Work out the finished part from the listing and answer in its coordinate system (mm). Face numbers are marked on the shaded views. A direction names the side the tool comes from. Coordinates: 2 decimals unless noted, no trailing zeros. Loops run counter-clockwise (first coordinate to the right, second up) from the corner with the lowest first, then second, coordinate; pieces in that order, holes last. Notation, with made-up numbers: M -27,75.25 L 7,75.25 A25 cw 7,112.25 Z; hole C 57.25,72 d4. An arc over 180 degrees is marked long. Write each question's results on one line, items separated by ' | '.
```python
from build123d import *

# Parameters (mm, degrees)
BOSS_EXTRUDE1_DEPTH     = 21
SKETCH3_R               = 14.5
BOSS_EXTRUDE2_DEPTH     = 16
CUT_EXTRUDE1_DEPTH      = 30.351320243
CUT_EXTRUDE1_DEPTH_BACK = 30.351320243
SKETCH4_R               = 5


with BuildPart() as part:
    # Sketch1 → Boss-Extrude1 (new body)
    with BuildSketch(Plane.XY):
        with BuildLine():
            Line((-8, 7.549834435), (-8, -7.549834435))
            ThreePointArc((-8, -7.549834435), (0, -11), (8, -7.549834435))
            Line((8, -7.549834435), (8, 7.549834435))
            ThreePointArc((8, 7.549834435), (0, 11), (-8, 7.549834435))
        make_face()
    extrude(amount=BOSS_EXTRUDE1_DEPTH)

    # Sketch3 → Boss-Extrude2 (add)
    with BuildSketch(Plane.XY):
        Circle(SKETCH3_R)
    extrude(amount=-BOSS_EXTRUDE2_DEPTH)

    # Sketch4 → Cut-Extrude1 (cut, two sides: drawn at the far end of the back side and taken through both)
    with BuildSketch(Plane(origin=(0, 0, 0), x_dir=(0, 0, -1), z_dir=(1, 0, 0)).offset(-CUT_EXTRUDE1_DEPTH_BACK)):
        with Locations((-11.179145377, 0)):
            Circle(SKETCH4_R)
    extrude(amount=CUT_EXTRUDE1_DEPTH + CUT_EXTRUDE1_DEPTH_BACK, mode=Mode.SUBTRACT)


solid = part.part
```
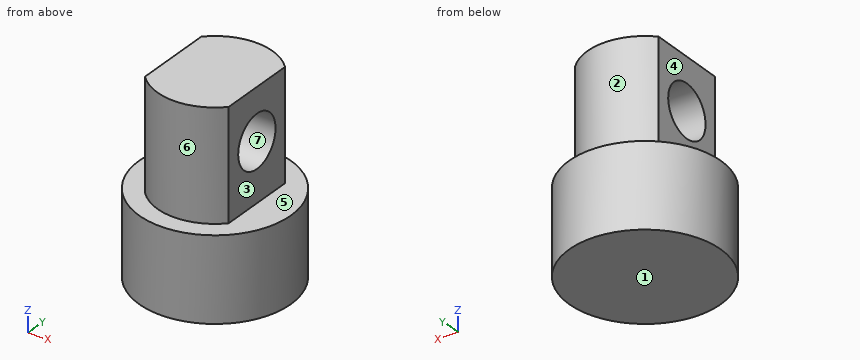
1) Find section D-D, the plane y = -4.25. Give the vertices of the cut face in (x, z).
Check result:
outline: M -13.86,-16 L 13.86,-16 L 13.86,0 L 8,0 L 8,8.55 L -8,8.55 L -8,0 L -13.86,0 Z; M -8,13.81 L 8,13.81 L 8,21 L -8,21 Z
2) For a pull along Z with two mould halves and no side action, classify the marked faces 5, 6 and 7 as released by +Z, released by -Z, zero draft, split by the parting line, or undercut.
Check result:
face 5: released by +Z | face 6: zero draft | face 7: undercut
3) Find section A-A, the plane y = 0. Give the vertices of the cut face in (x, z).
Check result:
outline: M -14.5,-16 L 14.5,-16 L 14.5,0 L 8,0 L 8,6.18 L -8,6.18 L -8,0 L -14.5,0 Z; M -8,16.18 L 8,16.18 L 8,21 L -8,21 Z
4) Find section C-C, the plane x = 0. Give the vertices of the cut face in (y, z).
Check result:
outline: M -14.5,-16 L 14.5,-16 L 14.5,0 L 11,0 L 11,21 L -11,21 L -11,0 L -14.5,0 Z; hole C 0,11.18 d10
5) Given pin 1 Ø16.5 at (y, z) = (1.5, 5.5) entering from -X; pin 2 Ø8 at (x, z) = (-10.5, -11.5) entering from +Y; pin 3 Ø13 at (y, z) = (0, 11.18) entering from +X; pin 4 Ø6 at (y, z) = (-6, 5.5) entering from -X, each flat-ended and moving along its own axis, determine where each tip first touches the part or whether it passes through.
Check result:
pin 1: x = -14.5 | pin 2: y = 12.96 | pin 3: x = 8 | pin 4: x = -8
6) Straight lines are drawn through the part: probe 1 along Z at (x, y) = (1.25, 0); probe 2 along Y at (x, z) = (0.25, 11); probe 3 along Y at (x, z) = (-0.5, -10.5). For each, find the intervals that lie inside material, in ascending order. Write a range as [from, to].
Check result:
probe 1: [-16, 6.18], [16.18, 21] | probe 2: [-11, -5], [5, 11] | probe 3: [-14.49, 14.49]
7) Which of the six approach directions +Z, -Z, +X, -X, +Y, -Y give full straight-line access (tool end or side, diameter ignored) to the marked faces 1, 2, 3 and 4?
Check result:
face 1: -Z, +X, -X, +Y, -Y | face 2: +Z, +Y | face 3: +Z, +X, +Y, -Y | face 4: +Z, -X, +Y, -Y
8) Find section B-B, the plane z = 15.5. Give the vertices of the cut face in (x, y), and give its area (3 significant figures).
Check result:
outline: M -8,-7.55 A11 ccw 8,-7.55 L 8,-2.52 L -8,-2.52 Z; M -8,2.52 L 8,2.52 L 8,7.55 A11 ccw -8,7.55 Z | area: 237 mm^2
